Part model, mm, in its own coordinate system. A direction names the side the tool comes from. Give positions to 0.01 mm unless a question says otherwise; leave off trailing zeros. Write each loop counter-clockwise with the first axis right and the second up, starting at its lowest first coordinate (ties: lowest second). Pieces come first, ordered by that corner, then holes. Notation, with made-up numbers: (-18.75, 68) - (30.25, 68) arc R18 cw to (30.25, 89) - close; hole circle Ø7 at (7.5, -39). An arc over 180 degrees is marked (long way). Answer in a Markdown table with one row per item. Add a question column.
1. Drop flat-ended pins along their axis: pin 1 Ø11.5 at (y, z) = (-15.5, -4.5) entering from -X; pin 2 Ø10 at (x, y) = (53.5, -3.5) entering from +Z; pin 3 Ø13.5 at (y, z) = (-16, -6.5) entering from +X; pin 4 Ø19 at (x, z) = (23.5, -1.5) entering from -Y. Give the stop position or say it passes through.
2. Which spindle directions (+Z, -Z, +X, -X, +Y, -Y) get a long thin tool onto all of the face, cutting with end or side? Do faces 1 (the cylindrical face through (11.717, -23.976, -8.619)), 2 (the flat face through (34, 3, 0)), 3 (the flat face through (62.5, -14, -8)), 4 (the flat face through (11, -15, -17)). Say none if no direction does.
3. Band-saw the part on C-C on y = -7. Write the cut outline in (x, z), plus the area to 3 significant figures.
4. Probe line 1 along Y through (x, z) = (61.5, -2); line 2 along Y through (x, z) = (66.5, -5); line 3 along Y through (x, z) = (58.5, -7.75). List the from-to ranges inside material, lowest first.
5. Band-saw the part on B-B on x = 36.5. Write the cut outline in (y, z), plus the area to 3 significant figures.
6. Pull direction Z, two halves, no side cores. Call faces 5 (the flat face through (0, -15, 2)), 6 (the flat face through (38.401, 11.339, -13.457)), 7 (the cylindrical face through (11.619, 14.227, 6.27)): released by +Z, released by -Z, zero draft, split by the parting line, or undercut.
7. Band-saw the part on A-A on y = -44. Write the cut outline in (x, z).
8. Band-saw the part on D-D on x = 25.5. Write the cut outline in (y, z).
```python
from build123d import *

# Parameters (mm, degrees)
SKETCH1_W           = 70
SKETCH1_H           = 30
SKETCH1_R           = 10.5
BOSS_EXTRUDE1_DEPTH = 4
SKETCH3_W           = 8.150987667
SKETCH3_H           = 10.43538234
SKETCH3_W_2         = 6.820916115
SKETCH3_H_2         = 20
BOSS_EXTRUDE2_DEPTH = 17
SKETCH4_R           = 1
CUT_EXTRUDE1_DEPTH  = 17
BOSS_EXTRUDE4_DEPTH = 3
BOSS_EXTRUDE5_DEPTH = 20
SKETCH10_R          = 2.75
CUT_EXTRUDE2_DEPTH  = 47.267747797
BOSS_EXTRUDE6_DEPTH = 3
BOSS_EXTRUDE7_DEPTH = 23


with BuildPart() as part:
    # Sketch1 → Boss-Extrude1 (new body)
    with BuildSketch(Plane.XY):
        with Locations((35, -15)):
            Rectangle(SKETCH1_W, SKETCH1_H)
        with Locations((35, -15)):
            Circle(SKETCH1_R, mode=Mode.SUBTRACT)
    extrude(amount=BOSS_EXTRUDE1_DEPTH)

    # Sketch3 → Boss-Extrude2 (add)
    with BuildSketch(Plane(origin=(0, 0, 0), x_dir=(-1, 0, 0), z_dir=(0, 0, -1))):
        with Locations((-58.424506167, -14.156074174)):
            Rectangle(SKETCH3_W, SKETCH3_H)
        with Locations((-10.910458058, -15)):
            Rectangle(SKETCH3_W_2, SKETCH3_H_2)
    extrude(amount=BOSS_EXTRUDE2_DEPTH)

    # Sketch4 → Cut-Extrude1 (cut)
    with BuildSketch(Plane(origin=(0, 0, -17), x_dir=(-1, 0, 0), z_dir=(0, 0, -1))):
        with Locations((-58.5, -14.289099526)):
            Circle(SKETCH4_R)
        with Locations((-11.5, -7)):
            Circle(SKETCH4_R)
        with Locations((-11.5, -23)):
            Circle(SKETCH4_R)
    extrude(amount=-CUT_EXTRUDE1_DEPTH, mode=Mode.SUBTRACT)

    # Sketch7 → Boss-Extrude4 (add)
    with BuildSketch(Plane(origin=(0, 0, 0), x_dir=(1, 0, 0), z_dir=(0, 1, 0))):
        Polygon((-4.630368757, -4), (65.950788783, -22.912164164), (73.197722046, 4.133758972), (2.616564506, 23.045923136), align=None)
    extrude(amount=BOSS_EXTRUDE4_DEPTH)

    # Sketch9 → Boss-Extrude5 (add)
    with BuildSketch(Plane(origin=(0, 3, 0), x_dir=(1, 0, 0), z_dir=(0, 1, 0))):
        Polygon((-4.630368757, -4), (65.950788783, -22.912164164), (66.943950204, -19.205635281), (-3.595092577, -0.136296695), align=None)
        Polygon((2.616564506, 23.045923136), (1.581288325, 19.182219831), (72.162445865, 0.270055667), (73.197722046, 4.133758972), align=None)
    extrude(amount=BOSS_EXTRUDE5_DEPTH)

    # Sketch10 → Cut-Extrude2 (cut, through all)
    with BuildSketch(Plane(origin=(5.936757371, 0, -22.156280139), x_dir=(-0.965925826, 0, -0.258819045), z_dir=(0.258819045, 0, -0.965925826))):
        with Locations((-53.953749554, 11.5)):
            Circle(SKETCH10_R)
        with Locations((-12.488324975, 11.5)):
            Circle(SKETCH10_R)
    extrude(amount=-CUT_EXTRUDE2_DEPTH, mode=Mode.SUBTRACT)

    # Sketch5 → Boss-Extrude6 (add)
    with BuildSketch(Plane.XZ.offset(30)):
        Polygon((-4.630368757, 4), (2.616564506, -23.045923136), (73.197722046, -4.133758972), (65.950788783, 22.912164164), align=None)
    extrude(amount=BOSS_EXTRUDE6_DEPTH)

    # Sketch6 → Boss-Extrude7 (add)
    with BuildSketch(Plane.XZ.offset(33)):
        Polygon((-4.630368757, 4), (-3.595092577, 0.136296695), (66.943950204, 19.205635281), (65.950788783, 22.912164164), align=None)
        Polygon((2.616564506, -23.045923136), (73.197722046, -4.133758972), (72.162445865, -0.270055667), (1.581288325, -19.182219831), align=None)
    extrude(amount=BOSS_EXTRUDE7_DEPTH)


solid = part.part
```
Values:
| question | item | result |
|---|---|---|
| 1 | pin 1 | stops at x = 0 |
| 1 | pin 2 | stops at z = 20.53 |
| 1 | pin 3 | stops at x = 70 |
| 1 | pin 4 | stops at y = -56 |
| 2 | face 1 | -Z |
| 2 | face 2 | +Y |
| 2 | face 3 | -Z, +X |
| 2 | face 4 | -Z, +X, -X |
| 3 | outline | (0, 0) - (7.5, 0) - (7.5, -17) - (10.5, -17) - (10.5, 0) - (12.5, 0) - (12.5, -17) - (14.32, -17) - (14.32, 0) - (28.2, 0) - (28.2, 4) - (0, 4) - close; (41.8, 0) - (70, 0) - (70, 4) - (41.8, 4) - close |
| 3 | area | 308 mm² |
| 4 | line 1 | y = -33 to -30, -19.37 to -8.94, 0 to 3 |
| 4 | line 2 | y = -56 to -30, 0 to 23 |
| 4 | line 3 | y = -56 to -30, -19.37 to -15.29, -13.29 to -8.94, 0 to 8.8, 14.2 to 23 |
| 5 | outline | (-56, -13.97) - (-30, -13.97) - (-30, 0) - (-25.39, 0) - (-25.39, 4) - (-30, 4) - (-30, 15.02) - (-56, 15.02) - (-56, 10.98) - (-33, 10.98) - (-33, -9.83) - (-56, -9.83) - close; (-4.61, 0) - (0, 0) - (0, -13.97) - (23, -13.97) - (23, -9.83) - (3, -9.83) - (3, 10.98) - (23, 10.98) - (23, 15.02) - (0, 15.02) - (0, 4) - (-4.61, 4) - close |
| 5 | area | 563 mm² |
| 6 | face 5 | zero draft |
| 6 | face 6 | released by -Z |
| 6 | face 7 | undercut |
| 7 | outline | (-4.63, 4) - (-3.6, 0.14) - (66.94, 19.21) - (65.95, 22.91) - close; (1.58, -19.18) - (2.62, -23.05) - (73.2, -4.13) - (72.16, -0.27) - close |
| 8 | outline | (-56, -16.91) - (-30, -16.91) - (-30, 0) - (-19.47, 0) - (-19.47, 4) - (-30, 4) - (-30, 12.07) - (-56, 12.07) - (-56, 8) - (-33, 8) - (-33, -12.77) - (-56, -12.77) - close; (-10.53, 0) - (0, 0) - (0, -16.91) - (23, -16.91) - (23, -12.77) - (3, -12.77) - (3, 8) - (23, 8) - (23, 12.07) - (0, 12.07) - (0, 4) - (-10.53, 4) - close |
